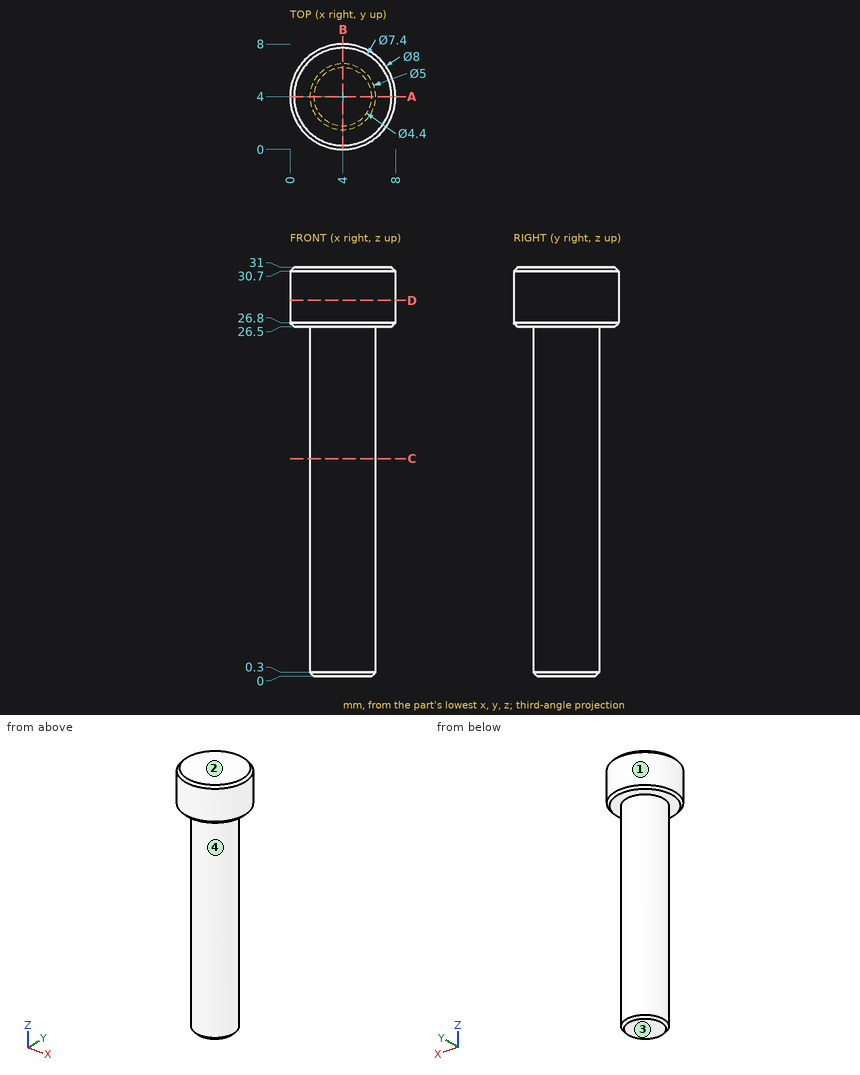
Here's the drawing with two shaded views (mm, measured from the low corner). I have some questions. A direction names the side the tool comes from. Coordinates: 2 decimals unless noted, no trailing zeros. Write each loop counter-clockwise with the first axis right and the second up, starting at its lowest first coordinate (ties: lowest second). Pieces come first, ordered by that corner, then holes. Notation, with made-up numbers: M 44,21 L 74,21 A11 cw 74,39 Z; hole C 80,0.25 d10. An arc over 180 degrees is marked long. Write item = value, one per line. Start each with the question number.
Q1. If we section it at A-A, the plane y = 4: Write out the boundary of the cut face in (x, z), then the cut area to 3 significant figures.
Q2. If we section it at D-D, the plane z = 28.5: Write out the boundary of the cut face in (x, y).
Q3. Thinking about a two-plate mould opening in Y: for the marked faces 1 and 2, which applies, released by +Y, released by -Y, zero draft, split by the parting line, or undercut?
Q4. If we section it at C-C, the plane z = 16.5: Write out the boundary of the cut face in (x, y), then the cut area to 3 significant figures.
Q5. On a 3-axis mill with a long thin cutter (end or side, diameter ignored), from which of +Z, -Z, +X, -X, +Y, -Y can I reach the whole of each face in a straight line? I mean the marked faces 3 and 4. Say none if no direction works.
Q6. I'm going to push flat-ended pins straight in: pin 1 (3 mm diameter, centred on y = 7, z = 10, fed in from -X); pin 2 (3 mm diameter, centred on x = 3.5, z = 6.5, fed in from -Y); pin 3 (1.5 mm diameter, centred on y = 7, z = 24, fed in from +X); pin 4 (2 mm diameter, centred on x = 4.5, y = 3, fed in from -Z). Where does each tip first touch, or does it pass through?
Q7. If I drill on L1, parallel to Z at x = 6.5, y = 3; L2, parallel to Y at x = 2.5, z = 23; L3, parallel to X at y = 5.25, z = 5.5, over which ranges is the centre line in solid material (lowest first)? Write a range as [from, to].
Check sheet entries:
q1.outline = M 0,26.8 L 0.3,26.5 L 1.5,26.5 L 1.5,0.3 L 1.8,0 L 6.2,0 L 6.5,0.3 L 6.5,26.5 L 7.7,26.5 L 8,26.8 L 8,30.7 L 7.7,31 L 0.3,31 L 0,30.7 Z
q1.area = 168 mm²
q2.outline = C 4,4 d8
q3.face_1 = split by the parting line
q3.face_2 = zero draft
q4.outline = C 4,4 d5
q4.area = 19.6 mm²
q5.face_3 = -Z, +X, -X, +Y, -Y
q5.face_4 = -Z
q6.pin_1 = 2
q6.pin_2 = 1.5
q6.pin_3 = 5.09
q6.pin_4 = 0
q7.L1 = [26.5, 31]
q7.L2 = [2, 6]
q7.L3 = [1.83, 6.17]
